The drawing under review shows one solid part. Ordinate dimensions are in mm from its lowest x, y, z. A direction names the side the tool comes from. Coordinates: 2 decimals unless noted, no trailing zeros. Order: outer loops, then holes, each group sorted by start corner. A loop starts at its lowest first (then second) coordinate and runs counter-clockwise, first axis right, second up. Notation, with made-up numbers: (26, -38) - (54, -38) arc R7 cw to (54, -34) - close; hole circle Ø4 at (33.5, 76.5). An arc over 180 degrees is marked (long way). Answer in a Markdown table with one row per item.
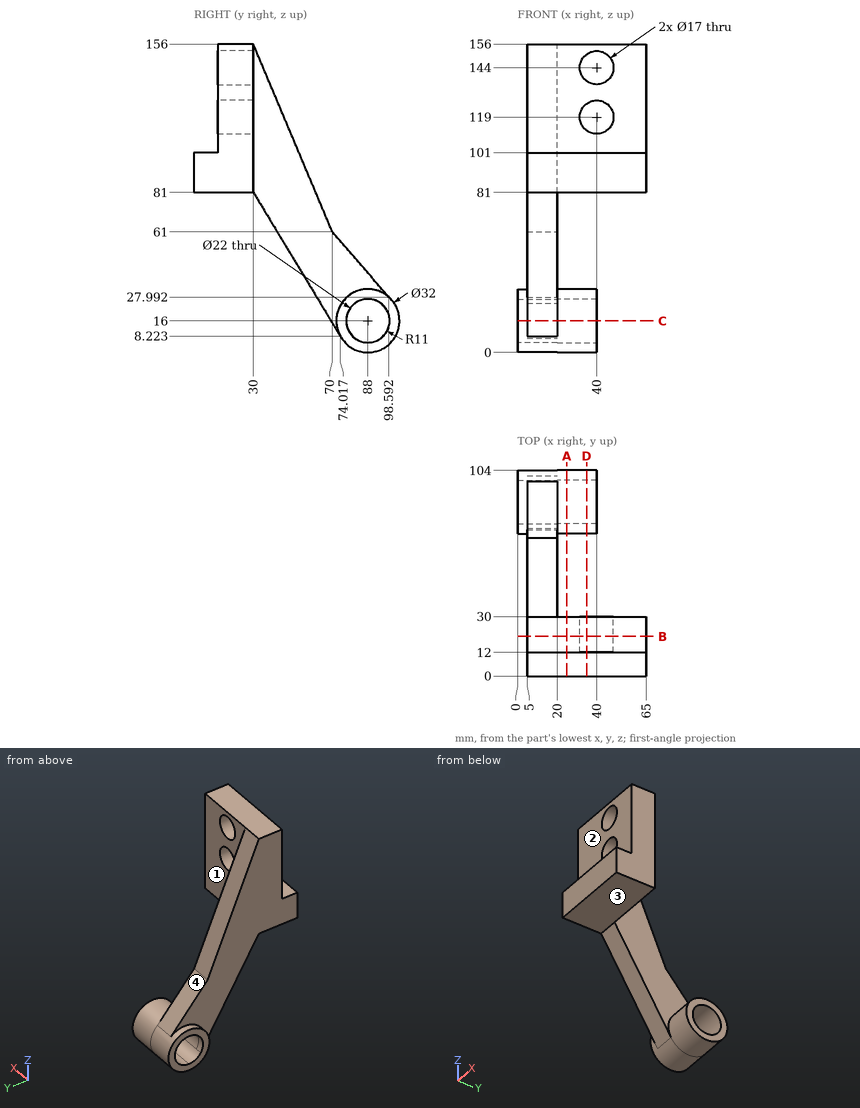
Item 1: Tool access review of the marked faces 1, 2, 3 and 4: name each direction out of +Z, -Z, +X, -X, +Y, -Y from which nothing blocks a thin tool from reaching the whole face with its end or side.
Check values:
| item | result |
|---|---|
| face 1 | +Z, -Z, +X, +Y |
| face 2 | +Z, +X, -X, -Y |
| face 3 | -Z, +X, -X, -Y |
| face 4 | +Z, +X, -X, +Y |
Item 2: We need section A-A, the plane x = 25. Write out the cut boundary in (y, z), then the cut area to 3 significant figures.
Check values:
| item | result |
|---|---|
| outline | (0, 81) - (30, 81) - (30, 156) - (12, 156) - (12, 101) - (0, 101) - close; circle Ø32 at (88, 16); hole circle Ø22 at (88, 16) |
| area | 2,010 mm^2 |
Item 3: We need section C-C, the plane z = 16. Write out the cut boundary in (x, y).
Check values:
| item | result |
|---|---|
| outline | (0, 72) - (5, 72) - (5, 69.31) - (20, 69.31) - (20, 72) - (40, 72) - (40, 77) - (0, 77) - close; (0, 99) - (40, 99) - (40, 104) - (0, 104) - close |
Item 4: Clearance check with flat-ended pins moving along their axes: pin 1 Ø5 at (x, z) = (44.5, 138) entering from -Y; pin 2 Ø10 at (x, z) = (40, 144) entering from -Y; pin 3 Ø20.5 at (y, z) = (57, 96) entering from +X; pin 4 Ø19.5 at (x, z) = (40, 119) entering from +Y. State where each tip first meets the part, or that it passes through.
Check values:
| item | result |
|---|---|
| pin 1 | y = 12 |
| pin 2 | through |
| pin 3 | x = 20 |
| pin 4 | y = 30 |
Item 5: We need section D-D, the plane x = 35. Write out the cut boundary in (y, z).
Check values:
| item | result |
|---|---|
| outline | (0, 81) - (30, 81) - (30, 112.13) - (12, 112.13) - (12, 101) - (0, 101) - close; (12, 125.87) - (30, 125.87) - (30, 137.13) - (12, 137.13) - close; (12, 150.87) - (30, 150.87) - (30, 156) - (12, 156) - close; circle Ø32 at (88, 16); hole circle Ø22 at (88, 16) |
Item 6: We need section B-B, the plane y = 20. Write out the cut boundary in (x, z).
Check values:
| item | result |
|---|---|
| outline | (5, 81) - (65, 81) - (65, 156) - (5, 156) - close; hole circle Ø17 at (40, 119); hole circle Ø17 at (40, 144) |
Item 7: To check wall thickness, follow line 1 (Y direction, x = 30, z = 16); line 2 (Z direction, x = 38, y = 14); line 3 (X direction, y = 22, z = 119). State the ranges of each line that lie inside material, in increasing order. Write a range as from..to.
Check values:
| item | result |
|---|---|
| line 1 | 72..77, 99..104 |
| line 2 | 81..110.74, 127.26..135.74, 152.26..156 |
| line 3 | 5..31.5, 48.5..65 |
